```python
from build123d import *

# Parameters (mm, degrees)
SKETCH1_R           = 15
SKETCH1_R_2         = 40
SKETCH1_R_3         = 20
BOSS_EXTRUDE1_DEPTH = 20
BOSS_EXTRUDE2_START = 80
SKETCH1_4_R         = 40
SKETCH1_4_R_2       = 20
BOSS_EXTRUDE2_DEPTH = 80
RIB14_REACH         = 140.564
SKETCH2_WALL_W      = 361.892855998
SKETCH2_WALL_H      = 10
CIRPATTERN1_COUNT   = 4


with BuildPart() as part:
    # Sketch1 → Boss-Extrude1 (new body)
    # profile 1 of 2: a face of its own
    with BuildSketch(Plane.XY):
        with BuildLine():
            Line((-50, 80), (50, 80))
            ThreePointArc((50, 80), (71.213203436, 71.213203436), (80, 50))
            Line((80, 50), (80, -50))
            ThreePointArc((80, -50), (71.213203436, -71.213203436), (50, -80))
            Line((50, -80), (-50, -80))
            ThreePointArc((-50, -80), (-71.213203436, -71.213203436), (-80, -50))
            Line((-80, -50), (-80, 50))
            ThreePointArc((-80, 50), (-71.213203436, 71.213203436), (-50, 80))
        make_face()
        with Locations((50, 50)):
            Circle(SKETCH1_R, mode=Mode.SUBTRACT)
        with Locations((-50, 50)):
            Circle(SKETCH1_R, mode=Mode.SUBTRACT)
        with Locations((-50, -50)):
            Circle(SKETCH1_R, mode=Mode.SUBTRACT)
        with Locations((50, -50)):
            Circle(SKETCH1_R, mode=Mode.SUBTRACT)
        Circle(SKETCH1_R_2, mode=Mode.SUBTRACT)
    # profile 2 of 2: a face of its own
    with BuildSketch(Plane.XY):
        Circle(SKETCH1_R_2)
        Circle(SKETCH1_R_3, mode=Mode.SUBTRACT)
    extrude(amount=-BOSS_EXTRUDE1_DEPTH)

    # Sketch1_4 → Boss-Extrude2 (add)
    with BuildSketch(Plane.XY.offset(BOSS_EXTRUDE2_START)):
        Circle(SKETCH1_4_R)
        Circle(SKETCH1_4_R_2, mode=Mode.SUBTRACT)
    extrude(amount=-BOSS_EXTRUDE2_DEPTH)

    # Sketch2 wall → Rib14 (add, up to next)
    with BuildSketch(Plane(origin=(57.5, 0, 37.5), x_dir=(0.422885465331, 0, -0.906183139995), z_dir=(-0.906183139995, 0, -0.422885465331)), mode=Mode.PRIVATE) as rib14_sk1:
        Rectangle(SKETCH2_WALL_W, SKETCH2_WALL_H)
    rib14_tool1 = extrude(rib14_sk1.sketch, amount=RIB14_REACH, mode=Mode.PRIVATE) - part.part
    rib14 = rib14_tool1.solids().sort_by_distance((57.5, 0, 37.5))[0]
    add(rib14)

    # CirPattern1: Rib14 ×4 about axis
    cirpattern1_axis = Axis((0, 0, 0), (0, 0, 1))
    for i in range(1, CIRPATTERN1_COUNT):
        add(rib14.rotate(cirpattern1_axis, i * 360 / CIRPATTERN1_COUNT))


solid = part.part
```
Work out the finished part from the listing and answer in its coordinate system (mm). A direction names the side the tool comes from. Give positions to 0.01 mm unless a question says otherwise; leave off trailing zeros. Write each loop counter-clockwise with the first axis right and the second up, starting at its lowest first coordinate (ties: lowest second). Pieces come first, ordered by that corner, then holes. Notation, with made-up numbers: (59, 64) -> (67, 64) arc R26 cw to (67, 102) -> close; hole circle Ø8 at (-16.75, 74.5). An arc over 180 degrees is marked (long way). Write item = value, one per line.
Q1. Section B-B on x = 0 is taken. Determine the outline of the cut face in (y, z).
Computed values:
outline = (-80, -20) -> (-20, -20) -> (-20, 80) -> (-40, 80) -> (-40, 75) -> (-75, 0) -> (-80, 0) -> close; (20, -20) -> (80, -20) -> (80, 0) -> (75, 0) -> (40, 75) -> (40, 80) -> (20, 80) -> close
Q2. Consider line 1 along Y through (x, z) = (-50, -14.75); line 2 along X through (y, z) = (-60, 19); line 3 along Y through (x, z) = (-1, 45). Determine where each line is inside the solid, lowest interval first.
Computed values:
line_1 = -80 to -65, -35 to 35, 65 to 80
line_2 = -5 to 5
line_3 = -54 to -19.97, 19.97 to 54
Q3. For a pull along X with two mould halves and no side action, classify faces 1 (the cylindrical face through (-61.056, 60.138, -9.86)), 2 (the flat face through (-9.4, 18.3, 80)), 3 (the flat face through (5, -50, 25)), 4 (the cylindrical face through (38.944, 60.138, -9.86)) as pulls with the +X half, pulls with the -X half, needs draft (parallel to the pull), parting line crosses it, or undercut.
Computed values:
face_1 = undercut
face_2 = needs draft
face_3 = pulls with the +X half
face_4 = undercut
Q4. Section A-A on z = 37.5 is taken. Determine the outline of the cut face in (x, y), and give its area (3 significant figures).
Computed values:
outline = (-57.5, -5) -> (-39.69, -5) arc R40 ccw to (-5, -39.69) -> (-5, -57.5) -> (5, -57.5) -> (5, -39.69) arc R40 ccw to (39.69, -5) -> (57.5, -5) -> (57.5, 5) -> (39.69, 5) arc R40 ccw to (5, 39.69) -> (5, 57.5) -> (-5, 57.5) -> (-5, 39.69) arc R40 ccw to (-39.69, 5) -> (-57.5, 5) -> close; hole circle Ø40 at (0, 0)
area = 4,470 mm^2
Q5. Flat-ended cylindrical pins translate along their axes: pin 1 Ø3 at (x, z) = (31, 27.5) entering from +Y; pin 2 Ø12 at (y, z) = (-6.5, 25.5) entering from -X; pin 3 Ø3 at (x, z) = (25.5, 4.5) entering from +Y; pin 4 Ø17.5 at (x, z) = (63, 48.5) entering from -Y. Find the tip coordinate at first contact, or state that the pin passes through.
Computed values:
pin_1 = 27.01
pin_2 = -65.81
pin_3 = 32
pin_4 = through
Q6. Section C-C on y = -8.5 is taken. Determine the outline of the cut face in (x, z).
Computed values:
outline = (-80, -20) -> (-18.1, -20) -> (-18.1, 80) -> (-39.09, 80) -> (-39.09, 0) -> (-80, 0) -> close; (18.1, -20) -> (80, -20) -> (80, 0) -> (39.09, 0) -> (39.09, 80) -> (18.1, 80) -> close
Q7. A tool of negligible diameter and unlimited length cuts with its end or side. For faces 5 (the flat face through (0.07, 57.096, 38.366)), 6 (the flat face through (-5, 50, 25)), 7 (the flat face through (-50, -5, 25)), from which of +Z, -Z, +X, -X, +Y, -Y can it reach the whole face along a straight path? Write none if from no direction.
Computed values:
face_5 = +Z, +X, -X, +Y
face_6 = +Z, -X, +Y
face_7 = +Z, -X, -Y
Q8. Section D-D on x = 54 is taken. Determine the outline of the cut face in (y, z), and give its area (3 significant figures).
Computed values:
outline = (-79.73, -20) -> (-64.46, -20) -> (-64.46, 0) -> (-79.73, 0) -> close; (-35.54, -20) -> (35.54, -20) -> (35.54, 0) -> (5, 0) -> (5, 45) -> (-5, 45) -> (-5, 0) -> (-35.54, 0) -> close; (64.46, -20) -> (79.73, -20) -> (79.73, 0) -> (64.46, 0) -> close
area = 2,480 mm^2
